Input: dimensioned drawing with shaded views. Units: mm. Origin: part minimum x, y, z. A direction names the side the tool comes from. Round coordinates to 2 decimals unless told otherwise and drop trailing zeros. Order: outer loops, then holes, each group sorted by start corner. A loop starts at its lowest first (then second) coordinate and runs counter-clockwise, first axis right, second up. Notation, with made-up numbers: M 22.25,87.5 L 41.25,87.5 A27 ccw 41.25,107.5 Z; hole C 29.25,-29.75 d10. An arc over 180 degrees is marked long. Use one line per item in the form item = value. Start each with the question number.
Q1. Section A-A (x = 17). Return the cut outline in (y, z), plus the area to 3 significant figures.
Q2. Section D-D (y = 10.5). Give the number of separate pieces and of enclosed holes in the cut face, plus the area to 3 significant figures.
Q3. Section B-B (y = 30). Return the cut outline in (x, z) (1 decimal).
Q4. Reachability of the marked faces 1 and 2 from +Z, -Z, +X, -X, +Y, -Y: full face, straight path, thin tool, end or side. Return the list, or none.
Q5. Section C-C (z = 27.5). Return the cut outline in (x, y), plus the area to 3 significant figures.
Q6. Material intervals for probe 1 along Y at (x, z) = (17, 68); probe 2 along Z at (x, y) = (20, 28.5); probe 3 along Y at (x, z) = (16.5, 62) (1 decimal), sorted ascending.
Q7. Contact query for flat-ended pins moving along their axis: pin 1 (12 mm diameter, centred on x = 14.5, z = 9.5, fed in from -Y); pin 2 (4 mm diameter, centred on y = 23.5, z = 50.5, fed in from -X) (1 decimal); pin 3 (4 mm diameter, centred on y = 10, z = 53, fed in from +X) (1 decimal). Output: stop coordinate, or through.
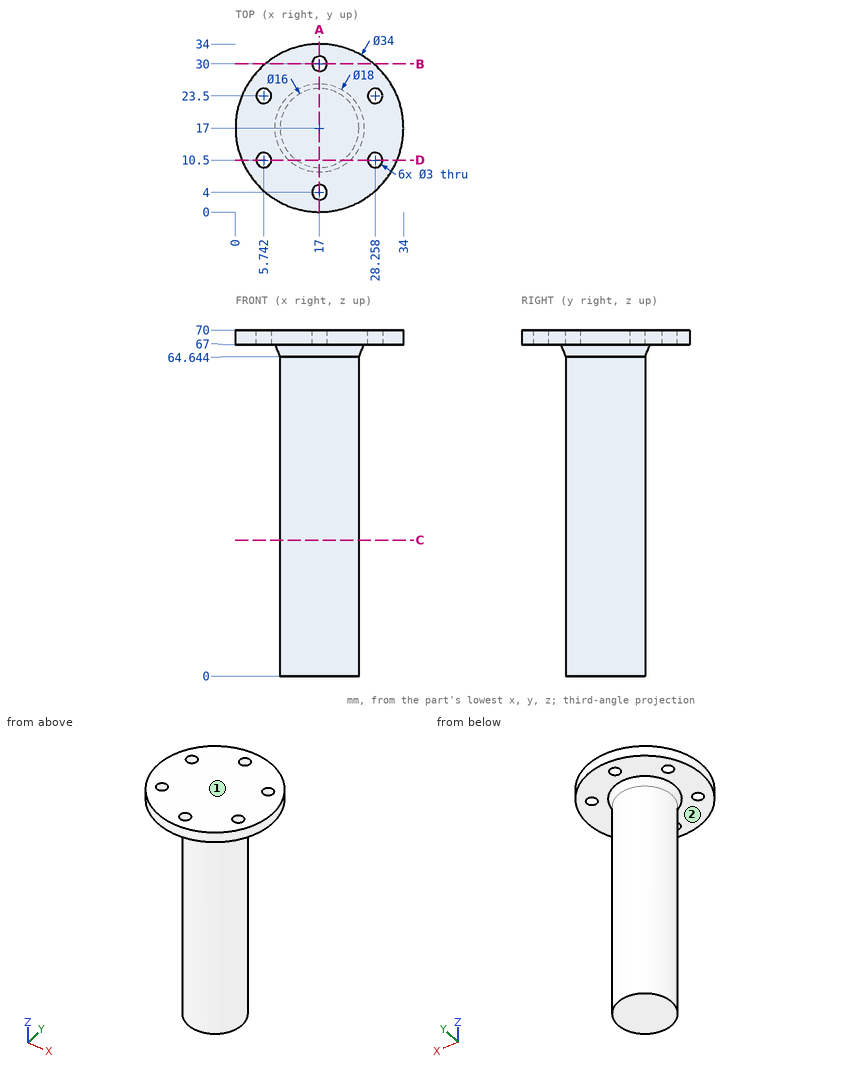
Results list:
q1.outline = M 0,67 L 2.5,67 L 2.5,70 L 0,70 Z; M 5.5,67 L 8,67 L 9,64.64 L 9,0 L 25,0 L 25,64.64 L 26,67 L 28.5,67 L 28.5,70 L 5.5,70 Z; M 31.5,67 L 34,67 L 34,70 L 31.5,70 Z
q1.area = 1,160 mm2
q2.separate_pieces = 3
q2.enclosed_holes = 0
q2.area = 705 mm2
q3.outline = M 6,67 L 15.5,67 L 15.5,70 L 6,70 Z; M 18.5,67 L 28,67 L 28,70 L 18.5,70 Z
q4.face_1 = +Z, +X, -X, +Y, -Y
q4.face_2 = -Z
q5.outline = C 17,17 d16
q5.area = 201 mm2
q6.probe_1 = 0 to 2.5, 5.5 to 28.5, 31.5 to 34
q6.probe_2 = 67 to 70
q6.probe_3 = 9 to 25
q7.pin_1 = 9
q7.pin_2 = 10.4
q7.pin_3 = 23.2
